Autodesk Fusion 360 part; units mm, degrees
sketch "Sketch1" plane through (0, 0, 0) normal (0, 1, 0) x (1, 0, 0)
  line L0 (0, 0) -> (0, -100)
  line L1 (12, -112) -> (12, -142)
  arc A0 (12, -112) -> (0, -100) centre (0, -112) ccw
  line L2 (12, -142) -> (24, -142)
  line L3 (0, 0) -> (12, 0)
  line L4 (12, 0) -> (12, -78)
  line L5 (24, -90) -> (72, -90)
  line L6 (32, -115) -> (58, -115)
  line L7 (24, -142) -> (24, -123)
  arc A1 (32, -115) -> (24, -123) centre (32, -123) ccw
  line L8 (66, -142) -> (66, -123)
  arc A2 (66, -123) -> (58, -115) centre (58, -123) ccw
  line L9 (66, -142) -> (72, -142)
  line L10 (72, -142) -> (72, -90)
  arc A3 (12, -78) -> (24, -90) centre (24, -78) ccw
  point P0 (12, -90)
  dimension "d1" = 100
  dimension "d2" = 24
  dimension "d4" = 142
  dimension "d6" = 12
  dimension "d7" = 90
  dimension "d8" = 25
  dimension "d9" = 8
  dimension "d10" = 42
  dimension "d11" = 8
  dimension "d12" = 6
  dimension "d13" = 12
extrude "Extrude1" add sketch "Sketch1" along normal blind 60
fillet "Fillet1" radius 12 2 edges at (18, 60, 142) (18, 0, 142)
fillet "Fillet2" radius 12 2 edges at (69, 0, 142) (69, 60, 142)
fillet "Fillet3" radius 12 2 edges at (6, 60, 0) (6, 0, 0)
sketch "Sketch2" plane through (0, 0, 0) normal (0, -1, 0) x (1, 0, 0)
  line L0 (0, 12) -> (12, 12)
  line L1 (12, 12) -> (12, 78)
  arc A0 (24, 90) -> (12, 78) centre (24, 78) ccw
  line L2 (24, 90) -> (72, 90)
  line L3 (72, 90) -> (72, 130)
  line L4 (72, 130) -> (66, 130)
  line L5 (66, 130) -> (66, 123)
  arc A1 (58, 115) -> (66, 123) centre (58, 123) ccw
  line L6 (58, 115) -> (32, 115)
  arc A2 (24, 123) -> (32, 115) centre (32, 123) ccw
  line L7 (24, 123) -> (24, 130)
  line L8 (24, 130) -> (12, 130)
  line L9 (12, 130) -> (12, 112)
  arc A3 (0, 100) -> (12, 112) centre (0, 112) ccw
  line L10 (0, 100) -> (0, 12)
  line L11 (60, 102) -> (72, 102)
  line L12 (72, 102) -> (72, 96)
  line L13 (72, 96) -> (60, 96)
  line L14 (60, 96) -> (60, 102)
  dimension "d22" = 6
  dimension "d23" = 12
  dimension "d24" = 12
extrude "Extrude2" cut sketch "Sketch2" against normal through all contours L3 L11 L12 L13 L14
sketch "Sketch3" plane through (72, 0, 0) normal (1, 0, 0) x (0, 1, 0)
  line L0 (0, 102) -> (60, 102)
  line L1 (60, 102) -> (60, 130)
  arc A0 (60, 130) -> (48, 142) centre (48, 130) ccw
  line L2 (48, 142) -> (12, 142)
  arc A1 (12, 142) -> (0, 130) centre (12, 130) ccw
  line L3 (0, 130) -> (0, 102)
  point P0 (30, 130)
hole "Hole1" at (72, 30, 130) direction (-1, 0, 0) diameter 12 depth 6 tip angle 118
sketch "Sketch4" plane through (12, 0, 0) normal (1, 0, 0) x (0, 1, 0)
  arc A0 (0, 12) -> (12, 0) centre (12, 12) ccw
  line L0 (12, 0) -> (48, 0)
  arc A1 (48, 0) -> (60, 12) centre (48, 12) ccw
  line L1 (60, 12) -> (60, 78)
  line L2 (60, 78) -> (0, 78)
  line L3 (0, 78) -> (0, 12)
  point P0 (15, 20)
  point P1 (45, 20)
  dimension "d30" = 15
  dimension "d31" = 15
  dimension "d32" = 20
hole "Hole2" at (12, 45, 20) at (12, 15, 20) direction (-1, 0, 0) diameter 10 depth 12 tip angle 118
sketch "Sketch5" plane through (12, 0, 0) normal (-1, 0, 0) x (0, -1, 0)
  arc A0 (0, 130) -> (-12, 142) centre (-12, 130) ccw
  line L0 (-12, 142) -> (-48, 142)
  arc A1 (-48, 142) -> (-60, 130) centre (-48, 130) ccw
  line L1 (-60, 130) -> (-60, 112)
  line L2 (-60, 112) -> (0, 112)
  line L3 (0, 112) -> (0, 130)
  point P0 (-45, 127)
  point P1 (-15, 127)
  dimension "d36" = 30
  dimension "d37" = 15
  dimension "d38" = 15
hole "Hole3" at (12, 45, 127) at (12, 15, 127) direction (1, 0, 0) diameter 10 depth 12 tip angle 118
For this review, take the finished solid that the model builds, in its own axes (mm). A direction names the side the tool comes from. Round coordinates to 2 decimals unless told otherwise and drop trailing zeros. Order: outer loops, then holes, each group sorted by start corner. A loop starts at its lowest first (then second) coordinate and runs counter-clockwise, first axis right, second up. Notation, with made-up numbers: (23.25, 69.25) -> (44.25, 69.25) arc R33 cw to (44.25, 101.25) -> close; hole circle Ø9 at (80.25, -2.75). An arc over 180 degrees is marked (long way). Use a Markdown table: item, result.
Item 1: For line 1 along Y through (x, z) = (21, 127); line 2 along Z through (x, y) = (38, 54); line 3 along Z through (x, y) = (18, 45), list the stretches that pass through material, from the lowest coordinate up. Write a range as [from, to].
Resolved:
| item | result |
|---|---|
| line 1 | y = [0, 10], [20, 40], [50, 60] |
| line 2 | z = [90, 115] |
| line 3 | z = [88.39, 122], [132, 142] |
Item 2: Take a section at B-B (z = 20). State the section outline as (x, y) points.
Resolved:
| item | result |
|---|---|
| outline | (0, 0) -> (12, 0) -> (12, 10) -> (0, 10) -> close; (0, 20) -> (12, 20) -> (12, 40) -> (0, 40) -> close; (0, 50) -> (12, 50) -> (12, 60) -> (0, 60) -> close |
Item 3: Machinability: for faces 5 (the cylindrical face through (18.08, 43.5, 131.77)), 6 (the cylindrical face through (8.39, 29.58, 103.42)), 7 (the flat face through (48, 30, 90)), which of the approach directions +Z, -Z, +X, -X, +Y, -Y give a long, thin tool a straight path to every point of the face, cutting with its end or side? Answer none if there is none.
Resolved:
| item | result |
|---|---|
| face 5 | -X |
| face 6 | +Z, -X, +Y, -Y |
| face 7 | -Z, +X, +Y, -Y |
Item 4: Take a section at A-A (y = 30). State the section outline as (x, z) points.
Resolved:
| item | result |
|---|---|
| outline | (0, 0) -> (12, 0) -> (12, 78) arc R12 cw to (24, 90) -> (72, 90) -> (72, 96) -> (60, 96) -> (60, 102) -> (72, 102) -> (72, 124) -> (66, 124) -> (66, 123) arc R8 cw to (58, 115) -> (32, 115) arc R8 cw to (24, 123) -> (24, 142) -> (12, 142) -> (12, 112) arc R12 cw to (0, 100) -> close; (66, 136) -> (72, 136) -> (72, 142) -> (66, 142) -> close |
Item 5: Draft analysis for pull direction X (two halves, no side actions). For faces 1 (the flat face through (0, 30, 49)), 2 (the flat face through (18, 30, 142)), 3 (the flat face through (24, 30, 133)), 4 (the cylindrical face through (26.281, 29.58, 117.406)), state which applies: +X half, -X half, draft (parallel to the pull), parting line (faces both ways), or undercut.
Resolved:
| item | result |
|---|---|
| face 1 | -X half |
| face 2 | draft |
| face 3 | undercut |
| face 4 | undercut |
Item 6: Take a section at C-C (x = 8). State the section outline as (y, z) points, plus the area to 3 significant figures.
Resolved:
| item | result |
|---|---|
| outline | (0, 12) arc R12 ccw to (12, 0) -> (48, 0) arc R12 ccw to (60, 12) -> (60, 103.06) -> (0, 103.06) -> close; hole circle Ø10 at (15, 20); hole circle Ø10 at (45, 20) |
| area | 5,960 mm² |
Item 7: For pin 1 (4 mm diameter, centred on x = 14.5, z = 24.5, fed in from +Y); pin 2 (1.5 mm diameter, centred on y = 13.5, z = 73.5, fed in from +X); pin 3 (9 mm diameter, centred on y = 43, z = 127, fed in from -X); pin 4 (13 mm diameter, centred on x = 66.5, y = 18.5, fed in from -Z), all flat-tipped, find the tip position at first contact; note any pin that passes through.
Resolved:
| item | result |
|---|---|
| pin 1 | passes through |
| pin 2 | stops at x = 12 |
| pin 3 | stops at x = 12 |
| pin 4 | stops at z = 90 |
Item 8: Take a section at D-D (y = 15). State the section outline as (x, z) points, plus the area to 3 significant figures.
Resolved:
| item | result |
|---|---|
| outline | (0, 0) -> (12, 0) -> (12, 15) -> (0, 15) -> close; (0, 25) -> (12, 25) -> (12, 78) arc R12 cw to (24, 90) -> (72, 90) -> (72, 96) -> (60, 96) -> (60, 102) -> (72, 102) -> (72, 142) -> (66, 142) -> (66, 123) arc R8 cw to (58, 115) -> (32, 115) arc R8 cw to (24.05, 122.09) -> (24, 122) -> (12, 122) -> (12, 112) arc R12 cw to (0, 100) -> close; (12, 132) -> (24, 132) -> (24, 142) -> (12, 142) -> close |
| area | 2,960 mm² |
